Source: CAD feature listing. Evaluate the final solid. Frame: model axes, mm. Face numbers are marked on the shaded views. A direction names the side the tool comes from. Coordinates: 2 decimals unless noted, no trailing zeros. Order: outer loops, then holes, each group sorted by start corner. A loop starts at its lowest first (then second) coordinate and runs counter-clockwise, first axis right, second up. Notation, with made-up numbers: (-17, 58) - (-2, 58) arc R22 cw to (-2, 81) - close; hole circle Ø11 at (-0.75, -15). An arc over 180 degrees is marked (long way). One line per question, with ' | ' between items. Start each with the question number.
(1) Draft query along Y for the marked faces 4, 5 and 6. Return one class per face: +Y half, -Y half, draft (parallel to the pull), parting line (faces both ways), or undercut.
(2) Section B-B (z = 0). Count the separate pieces of the cut face and the enclosed holes in it, then the cut area to 3 significant figures.
(3) Contact query for flat-ended pins moving along their axis: P1, Ø1.6, axis at x = 5.79, z = -6, coming from the +Y side; P2, Ø2, axis at y = -5, z = 0, coming from the -X side; P3, Ø3, axis at x = -1, y = -8.5, coming from the -Z side. Output: stop coordinate, or through.
(4) Section D-D (y = 2.5). Return the cut outline in (x, z), then the cut area to 3 significant figures.
(5) Section A-A (x = 5.79). Return the cut outline in (y, z), then the cut area to 3 significant figures.
(6) Line query: line 1 along X through (y, z) = (18.5, 0); line 2 along Y through (x, z) = (12.5, 3.25); line 3 along Z through (x, y) = (3.5, -6.5). Output: solid intervals per line, ascending.
(7) Section C-C (x = -2.5). Return the cut outline in (y, z), then the cut area to 3 significant figures.
(8) Access query for the marked faces 1, 2 and 3. Directions: +Z, -Z, +X, -X, +Y, -Y. A direction counts if a zero-diameter tool reaches every point of the face in a straight line with its end or side. Return the directions, or none.
from build123d import *

# Parameters (mm, degrees)
BOSS_EXTRUDE1_DEPTH      = 6
BOSS_EXTRUDE1_DEPTH_BACK = 6
SKETCH1_W                = 23
SKETCH1_H                = 27.5
SKETCH4_R                = 4.5
BOSS_EXTRUDE2_DEPTH      = 4.4
SKETCH5_R                = 9
BOSS_EXTRUDE3_DEPTH      = 1.2
SKETCH6_R                = 1
CUT_EXTRUDE1_DEPTH       = 1.2
SKETCH7_W                = 12
SKETCH7_H                = 1.5
BOSS_EXTRUDE4_DEPTH      = 4.5
SKETCH8_W                = 12
SKETCH8_H                = 5
BOSS_EXTRUDE5_DEPTH      = 3


with BuildPart() as part:
    # Sketch1 → Boss-Extrude1 (new, two sides: drawn at the far end of the back side and taken through both)
    with BuildSketch(Plane.XY.offset(-BOSS_EXTRUDE1_DEPTH_BACK)):
        Rectangle(SKETCH1_W, SKETCH1_H)
    extrude(amount=BOSS_EXTRUDE1_DEPTH + BOSS_EXTRUDE1_DEPTH_BACK)

    # Sketch4 → Boss-Extrude2 (add)
    with BuildSketch(Plane(origin=(0, 13.75, 0), x_dir=(1, 0, 0), z_dir=(0, 1, 0))):
        with Locations(Location((5.79, 0, 0), (0, 0, 270))):
            Circle(SKETCH4_R)
    extrude(amount=BOSS_EXTRUDE2_DEPTH)

    # Sketch5 → Boss-Extrude3 (add)
    with BuildSketch(Plane(origin=(0, 18.15, 0), x_dir=(1, 0, 0), z_dir=(0, 1, 0))):
        with Locations(Location((5.79, 0, 0), (0, 0, 270))):
            Circle(SKETCH5_R)
    extrude(amount=BOSS_EXTRUDE3_DEPTH)

    # Sketch6 → Cut-Extrude1 (cut)
    with BuildSketch(Plane(origin=(0, 19.35, 0), x_dir=(1, 0, 0), z_dir=(0, 1, 0))):
        with Locations(Location((5.79, 6, 0), (0, 0, 270))):
            Circle(SKETCH6_R)
        with Locations(Location((10.032640687, 4.242640687, 0), (0, 0, 270))):
            Circle(SKETCH6_R)
        with Locations(Location((11.79, 0, 0), (0, 0, 270))):
            Circle(SKETCH6_R)
        with Locations(Location((10.032640687, -4.242640687, 0), (0, 0, 270))):
            Circle(SKETCH6_R)
        with Locations(Location((5.79, -6, 0), (0, 0, 270))):
            Circle(SKETCH6_R)
        with Locations(Location((1.547359313, -4.242640687, 0), (0, 0, 270))):
            Circle(SKETCH6_R)
        with Locations(Location((-0.21, 0, 0), (0, 0, 270))):
            Circle(SKETCH6_R)
        with Locations(Location((1.547359313, 4.242640687, 0), (0, 0, 270))):
            Circle(SKETCH6_R)
    extrude(amount=-CUT_EXTRUDE1_DEPTH, mode=Mode.SUBTRACT)

    # Sketch7 → Boss-Extrude4 (add)
    with BuildSketch(Plane.ZY.offset(11.5)):
        with Locations((0, 7.5)):
            Rectangle(SKETCH7_W, SKETCH7_H)
    boss_extrude4 = extrude(amount=BOSS_EXTRUDE4_DEPTH)

    # Mirror1: Boss-Extrude4 across plane
    add(boss_extrude4.mirror(Plane(origin=(0, 0, 0), x_dir=(0, 0, 1), z_dir=(1, 0, 0))))

    # Sketch8 → Boss-Extrude5 (add)
    with BuildSketch(Plane(origin=(11.5, 0, 0), x_dir=(0, 0, -1), z_dir=(1, 0, 0))):
        with Locations((0, -5.75)):
            Rectangle(SKETCH8_W, SKETCH8_H)
    extrude(amount=BOSS_EXTRUDE5_DEPTH)


solid = part.part
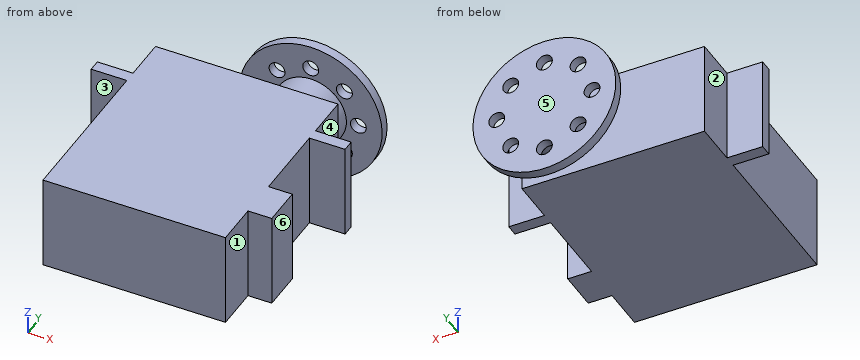
Response values:
1) face 4: undercut | face 5: +Y half | face 6: draft
2) separate pieces: 3 | enclosed holes: 0 | area: 717 mm²
3) P1: stops at y = 13.75 | P2: stops at x = -11.5 | P3: stops at z = -6
4) outline: (-11.5, -6) - (11.5, -6) - (11.5, 6) - (-11.5, 6) - close | area: 276 mm²
5) outline: (-13.75, -6) - (13.75, -6) - (13.75, -4.5) - (18.15, -4.5) - (18.15, -5) - (19.35, -5) - (19.35, 5) - (18.15, 5) - (18.15, 4.5) - (13.75, 4.5) - (13.75, 6) - (-13.75, 6) - close; (18.15, -9) - (19.35, -9) - (19.35, -7) - (18.15, -7) - close; (18.15, 7) - (19.35, 7) - (19.35, 9) - (18.15, 9) - close | area: 386 mm²
6) line 1: x = -3.21 to -1.21, 0.79 to 10.79, 12.79 to 14.79 | line 2: y = -8.25 to -3.25, 6.75 to 8.25, 18.15 to 19.35 | line 3: z = -6 to 6
7) outline: (-13.75, -6) - (13.75, -6) - (13.75, 6) - (-13.75, 6) - close; (18.15, -3.5) - (19.35, -3.5) - (19.35, 3.5) - (18.15, 3.5) - close | area: 338 mm²
8) face 1: +Z, -Z, +X, -Y | face 2: +Z, -Z, -X, +Y | face 3: +Z, -Z, -X, -Y
